Source: CAD feature listing. Evaluate the final solid. Frame: model axes, mm. A direction names the side the tool comes from. Give positions to 0.01 mm unless a question says otherwise; leave off trailing zeros. Loops run counter-clockwise (first coordinate to the right, second up) from the corner with the lowest first, then second, coordinate; pieces in that order, holes last. Notation, with made-up numbers: M -37,-12 L -14,-12 A25 cw -14,0 Z; hole C 36,16 d3. An arc over 180 degrees is marked long. Answer in a Markdown table with one row per item.
```python
from build123d import *

# Parameters (mm, degrees)
CHAMFER1_SIZE = 3.175


with BuildPart() as part:
    # Sketch1 → Revolve1 (revolve)
    with BuildSketch(Plane.XY):
        with BuildLine():
            Line((0, 27.305), (0, 9.525))
            Line((0, 9.525), (23.495, 9.525))
            Line((23.495, 9.525), (23.495, 27.305))
            Line((23.495, 27.305), (12.7, 27.305))
            Line((12.7, 27.305), (12.7, 24.13))
            ThreePointArc((12.7, 24.13), (10.16, 21.59), (7.62, 24.13))
            Line((7.62, 24.13), (7.62, 27.305))
            Line((7.62, 27.305), (0, 27.305))
        make_face()
    revolve(axis=Axis((0, 0, 0), (1, 0, 0)))

    # Chamfer1
    chamfer1_edges = [part.edges().sort_by_distance(p)[0] for p in [
        (0, -27.305, 0),
    ]]
    chamfer(chamfer1_edges, length=CHAMFER1_SIZE)


solid = part.part
```
Q1. Ray query, probe 1 along X at (y, z) = (-22, -9.5) (3 decimals); probe 2 along Z at (x, y) = (17.25, 0) (3 decimals); probe 3 along Z at (x, y) = (11.75, -5). Return the intervals inside material, ascending. Write a range as from..to.
Values follow:
| item | result |
|---|---|
| probe 1 | 0..7.625, 12.695..23.495 |
| probe 2 | -27.305..-9.525, 9.525..27.305 |
| probe 3 | -21.58..-8.11, 8.11..21.58 |
Q2. Section query C-C (x = 2). Output: boundary loops of the cut face in (y, z) (3 decimals), plus the area to 3 significant figures.
Values follow:
| item | result |
|---|---|
| outline | C 0,0 d52.26; hole C 0,0 d19.05 |
| area | 1,860 mm^2 |
Q3. Contact query for flat-ended pins moving along their axis: pin 1 Ø4 at (x, z) = (15.5, -21.5) entering from +Y; pin 2 Ø6 at (x, z) = (3, 15) entering from -Y; pin 3 Ø12 at (x, y) = (15.5, 15.5) entering from -Z; pin 4 Ø10 at (y, z) = (-4.5, -11) entering from -X. Output: stop coordinate, or through.
Values follow:
| item | result |
|---|---|
| pin 1 | y = 19.11 |
| pin 2 | y = -24.52 |
| pin 3 | z = -25.6 |
| pin 4 | x = 0 |
Q4. Mould query, pull axis X, two halves, no side actions, for faces 3 (the conical face through (0.2, -5.27, -23.75)), 4 (the cylindrical face through (5.366, -3.555, 27.073)), 5 (the flat face through (12.7, 14, -20)). Classes: +X half, -X half, draft (parallel to the pull), parting line (faces both ways), or undercut.
Values follow:
| item | result |
|---|---|
| face 3 | -X half |
| face 4 | draft |
| face 5 | undercut |
Q5. Section query D-D (x = 6). Output: boundary loops of the cut face in (y, z) (3 decimals), plus the area to 3 significant figures.
Values follow:
| item | result |
|---|---|
| outline | C 0,0 d54.61; hole C 0,0 d19.05 |
| area | 2,060 mm^2 |
Q6. Reachability of faces 1 (the flat face through (7.62, -14, -20)), 2 (the flat face through (0, 0, -10)) from +Z, -Z, +X, -X, +Y, -Y: full face, straight path, thin tool, end or side. Return the list, or none.
Values follow:
| item | result |
|---|---|
| face 1 | none |
| face 2 | +Z, -Z, -X, +Y, -Y |
Q7. Section query A-A (y = 0). Output: boundary loops of the cut face in (x, z) (3 decimals), plus the area to 3 significant figures.
Values follow:
| item | result |
|---|---|
| outline | M 0,-24.13 L 3.175,-27.305 L 7.62,-27.305 L 7.62,-24.13 A2.54 cw 12.7,-24.13 L 12.7,-27.305 L 23.495,-27.305 L 23.495,-9.525 L 0,-9.525 Z; M 0,9.525 L 23.495,9.525 L 23.495,27.305 L 12.7,27.305 L 12.7,24.13 A2.54 cw 7.62,24.13 L 7.62,27.305 L 3.175,27.305 L 0,24.13 Z |
| area | 773 mm^2 |
